Autodesk Inventor part; units mm, degrees
ref_plane "YZ Plane" through (0, 0, 0) normal (1, 0, 0) x (0, 1, 0)
ref_plane "XZ Plane" through (0, 0, 0) normal (0, 1, 0) x (-1, 0, 0)
ref_plane "XY Plane" through (0, 0, 0) normal (0, 0, 1) x (1, 0, 0)
sketch "Sketch1" plane through (0, 0, 0) normal (1, 0, 0) x (0, 1, 0)
  circle A0 centre (0, 0) radius 25.4
  dimension "d0" = 50.8
extrude "Extrusion1" add sketch "Sketch1" along normal blind 228.6
sketch "Sketch2" plane through (228.6, 0, 0) normal (1, 0, 0) x (0, 0, -1)
  circle A0 centre (0, 0) radius 6.35
  dimension "d3" = 12.7
extrude "Extrusion2" add sketch "Sketch2" along normal blind 19.05
chamfer "Chamfer1" distance 1.27 angle 45 1 edges at (247.65, 0, 6.35)
sketch "Sketch3" plane through (0, 0, 0) normal (-1, 0, 0) x (0, 0, 1)
  circle A0 centre (0, 0) radius 6.35
  circle A1 centre (0, 0) radius 6.35
extrude "Extrusion3" add sketch "Sketch3" along normal blind 19.05
chamfer "Chamfer2" distance 1.27 angle 45 1 edges at (-19.05, 0, -6.35)
properties part number "Roller Pin"
Verification items for the finished model (mm, model axes). A direction names the side the tool comes from. Coordinates: 2 decimals unless noted, no trailing zeros. Order: outer loops, then holes, each group sorted by start corner. A loop starts at its lowest first (then second) coordinate and runs counter-clockwise, first axis right, second up. Notation, with made-up numbers: (44, 83.5) -> (60, 83.5) arc R13 cw to (60, 87.5) -> close; hole circle Ø9 at (34.5, 22.5). An arc over 180 degrees is marked (long way). Put each result on its own line as item: value. Start each with the question number.
1) Go/stop test with flat-tipped pins: pin 1 (3 mm diameter, centred on x = 200.5, z = -12, fed in from -Y); pin 2 (1.5 mm diameter, centred on y = 10.5, z = 12.5, fed in from -X); pin 3 (12 mm diameter, centred on x = 59.5, y = -17.5, fed in from +Z). Record where each tip stops, or that it passes through.
2) Cross-section at D-D (y = -15). Enter the section's corners in (x, z).
3) Material ranges on L1, parallel to X at y = 12, z = 5.5; L2, parallel to Y at x = 235, z = -0.5; L3, parallel to Z at x = 106, y = 2.5, recorded low to high.
4) Cross-section at A-A (z = 0). Enter the section's corners in (x, y).
5) Tool access check on faces 1 (the flat face through (0, 5, -5)), 2 (the flat face through (247.65, 0, 0)), 3 (the flat face through (228.6, 5, -5)). Record the directions out of +Z, -Z, +X, -X, +Y, -Y that give a thin tool (end or side, any length) a straight path to the whole face; none if there is none.
6) Cross-section at C-C (x = 161). Enter the section's corners in (y, z), plus the area to 3 significant figures.
Geometry check:
1. pin 1: stops at y = -23.13
1. pin 2: stops at x = 0
1. pin 3: stops at z = 22.65
2. outline: (0, -20.5) -> (228.6, -20.5) -> (228.6, 20.5) -> (0, 20.5) -> close
3. L1: x = 0 to 228.6
3. L2: y = -6.33 to 6.33
3. L3: z = -25.28 to 25.28
4. outline: (-19.05, -5.08) -> (-17.78, -6.35) -> (0, -6.35) -> (0, -25.4) -> (228.6, -25.4) -> (228.6, -6.35) -> (246.38, -6.35) -> (247.65, -5.08) -> (247.65, 5.08) -> (246.38, 6.35) -> (228.6, 6.35) -> (228.6, 25.4) -> (0, 25.4) -> (0, 6.35) -> (-17.78, 6.35) -> (-19.05, 5.08) -> close
5. face 1: -X
5. face 2: +Z, -Z, +X, +Y, -Y
5. face 3: +X
6. outline: circle Ø50.8 at (0, 0)
6. area: 2,030 mm^2
